The model under review builds one solid part; all positions refer to its coordinate system, in mm. A direction names the side the tool comes from. Round coordinates to 2 decimals unless told otherwise and drop trailing zeros. Write each loop counter-clockwise with the first axis right and the second up, starting at its lowest first coordinate (ties: lowest second). Pieces come first, ordered by that corner, then holes. Notation, with made-up numbers: M 6.5,43.5 L 38.5,43.5 A11 cw 38.5,60.5 Z; hole C 67,38 d2. An arc over 180 degrees is marked long. One line per item, written item: value. Start each with the question number.
1) Take a section at A-A, the plane x = 21. Write out the cut boundary in (y, z), and give its area (3 significant figures).
2) Mouldability with a two-part tool opening along Z and no side actions: class faces 1 (the face through (12.878, -8.153, 10.633)), 2 (the face through (12.88, 13.85, 1.82)), 3 (the face through (50.44, 6.2, 1.38)) as +Z half, -Z half, draft (parallel to the pull), parting line (faces both ways), or undercut.
3) Wall thickness on probe 1 along Y at (x, z) = (5.75, 0); probe 2 along Y at (x, z) = (16, -8); probe 3 along Z at (x, y) = (53, 5.5): over which ranges is each line inside the solid? List them lowest first.
4) For P1, Ø1.5, axis at x = 14, z = -9.5, coming from the -Y side; P2, Ø5, axis at x = 70.5, y = 5.5, coming from the -Z side; P3, Ø1.5, axis at x = 77.5, y = -3, coming from the +Z side, all flat-tipped, find the tip position at first contact; note any pin that passes through.
5) Tool access review of faces 4 (the face through (74.237, -0.922, -7.023)), 5 (the face through (76.2, 0, 0)): name each direction out of +Z, -Z, +X, -X, +Y, -Y from which nothing blocks a thin tool from reaching the whole face with its end or side.
6) Take a section at B-B, the plane x = 77.5. Write out the cut boundary in (y, z).
Autodesk Fusion 360 part; units mm, degrees
sketch "Sketch1" plane through (0, 0, 0) normal (0, 0, 1) x (1, 0, 0)
  circle A0 centre (0, 0) radius 13.97
  circle A1 centre (0, 0) radius 13.3922
  dimension "d1" = 27.94
  dimension "d2" = 26.7843
sketch "Sketch2" plane through (0, 0, 0) normal (0, 0, 1) x (1, 0, 0)
  line L0 (35.56, 6.35) -> (80.4496, 0.4456)
  line L1 (80.4496, 0.4456) -> (35.56, 1.27)
  line L2 (35.56, 1.27) -> (35.56, 6.35)
  dimension "d5" = 45.2762
sketch "Sketch3" plane through (0, 0, 0) normal (0, 0, 1) x (1, 0, 0)
  line L0 (25.4, 0) -> (25.4, 13.97)
  line L1 (25.4, 13.97) -> (124.46, 0)
  line L2 (124.46, 0) -> (25.4, 0)
  dimension "d7" = 13.97
revolve "Revolve2" add sketch "Sketch3" angle 360 about axis through (124.46, 0, 0) along (-1, 0, 0)
sketch "Sketch4" plane through (0, 0, 0) normal (1, 0, 0) x (0, 0, -1)
  circle A0 centre (0, 0) radius 6.35
  dimension "d9" = 12.7
extrude "Extrude2" cut sketch "Sketch4" along normal blind 76.2
sketch "Sketch5" plane through (0, 0, 0) normal (1, 0, 0) x (0, 0, -1)
  circle A0 centre (0, 0) radius 13.97
cylinder "CylinderPrimitive1" add diameter 27.94 height 25.4 placed x (0, 0, -1) y (0, 1, 0) z (1, 0, 0) at (0, 0, 0)
cylinder "CylinderPrimitive2" cut diameter 26.797 height 25.4 placed x (0, 0, -1) y (0, 1, 0) z (1, 0, 0) at (0, 0, 0)
sketch "Sketch7" plane through (0, 0, 0) normal (1, 0, 0) x (0, 0, -1)
thread "Thread2"
hole "Hole1" at (74.2525, 7.0806, 0) direction (-0.1396, -0.9902, 0) diameter 2.54 depth 3.81 tip angle 118
Checked values:
1. outline: C 0,0 d27.94; hole C 0,0 d26.8
1. area: 49.1 mm2
2. face 1: undercut
2. face 2: parting line
2. face 3: undercut
3. probe 1: y = -13.97 to -13.4, 13.4 to 13.97
3. probe 2: y = -11.45 to -10.75, 10.75 to 11.45
3. probe 3: z = -8.44 to -3.17, 3.17 to 8.44
4. P1: stops at y = -10.89
4. P2: stops at z = -7.06
4. P3: stops at z = 6.25
5. face 4: +X
5. face 5: -X
6. outline: C 0,0 d13.25
